Input: part model. Units: mm. Frame: model coordinates. A direction names the side the tool comes from. Coordinates: 2 decimals unless noted, no trailing zeros. Loops run counter-clockwise (first coordinate to the right, second up) from the corner with the lowest first, then second, coordinate; pieces in that order, holes last. Notation, with made-up numbers: (-28, 66) -> (-10, 66) arc R29 ccw to (-10, 94) -> close; hole circle Ø3 at (73.25, 49.25). An arc over 180 degrees is marked (long way). Put each result on its own line as item: value. Start each with the question number.
1) Cut plane A-A (z = 12). Return the cut outline in (x, y), plus the area to 3 significant figures.
2) Material intervals for L1, parallel to X at y = 8, z = 330; L2, parallel to X at y = 0.75, z = 201.5; L3, parallel to Y at x = 1, z = 164, sorted ascending.
3) Pull-direction query (X, two-part tool) for faces 1 (the flat face through (30, 0, 12)), 2 (the flat face through (0, 0, 0)), 3 (the cylindrical face through (11.923, 3.755, 197.2)), 4 (the flat face through (-30, 0, 12)); classes: pulls with the +X half, pulls with the -X half, needs draft (parallel to the pull), parting line crosses it, or undercut.
4) Contact query for flat-ended pins moving along their axis: P1, Ø4, axis at x = 10, y = -3, coming from the +Z side; P2, Ø1.5, axis at x = -10, y = 8, coming from the +Z side; P3, Ø2, axis at y = 3, z = 262.5, coming from the -X side. Output: stop coordinate, or through.
5) Cut plane D-D (z = 99). Return the cut outline in (x, y).
6) Set-up query: faces 5 (the cylindrical face through (19.95, -1.73, 4.19)), 6 (the cylindrical face through (-19.66, 7.39, 8.94)), 7 (the flat face through (-0.2, -0.2, 387.7)). Return all of +Z, -Z, +X, -X, +Y, -Y with unobstructed straight access to the full face (end or side cutting, diameter ignored); none if empty.
7) Cut plane B-B (y = 0). Return the cut outline in (x, z).
8) Cut plane C-C (x = 25.5). Return the cut outline in (y, z).
from build123d import *

# Parameters (mm, degrees)
F0_R          = 12.5
F1_DEPTH      = 400
F2_R          = 8
F3_DEPTH      = 30
F5_DEPTH      = 30.0010001
F5_DEPTH_BACK = 30.0010001


with BuildPart() as f1:
    # F0 (on Top) → F1 (new body)
    with BuildSketch(Plane.XY):
        Circle(F0_R)
    extrude(amount=F1_DEPTH)

    # F2 (on Right) → F3 (join, symmetric)
    with BuildSketch(Plane.YZ):
        with Locations((0, 12)):
            Circle(F2_R)
    extrude(amount=F3_DEPTH, both=True)

    # F4 (on Right) → F5 (cut, two sides)
    with BuildSketch(Plane.YZ) as f5_sk:
        Polygon((12.5, 400), (-12.5, 400), (12.5, 375), align=None)
    extrude(amount=-F5_DEPTH, mode=Mode.SUBTRACT)
    extrude(f5_sk.sketch, amount=F5_DEPTH_BACK, mode=Mode.SUBTRACT)


solid = f1.part
Results found:
1. outline: (-30, -8) -> (-9.6, -8) arc R12.5 ccw to (9.6, -8) -> (30, -8) -> (30, 8) -> (9.6, 8) arc R12.5 ccw to (-9.6, 8) -> (-30, 8) -> close
1. area: 1,080 mm2
2. L1: x = -9.6 to 9.6
2. L2: x = -12.48 to 12.48
2. L3: y = -12.46 to 12.46
3. face 1: pulls with the +X half
3. face 2: needs draft
3. face 3: parting line crosses it
3. face 4: pulls with the -X half
4. P1: stops at z = 392.5
4. P2: stops at z = 380.25
4. P3: stops at x = -12.34
5. outline: circle Ø25 at (0, 0)
6. face 5: +X
6. face 6: -X
6. face 7: +Z, +X, -X, +Y
7. outline: (-30, 4) -> (-12.5, 4) -> (-12.5, 0) -> (12.5, 0) -> (12.5, 4) -> (30, 4) -> (30, 20) -> (12.5, 20) -> (12.5, 387.5) -> (-12.5, 387.5) -> (-12.5, 20) -> (-30, 20) -> close
8. outline: circle Ø16 at (0, 12)
